CAD build for the part. Positions are in the model's coordinates, mm. Face numbers are marked on the shaded views. A direction names the side the tool comes from. Coordinates: 2 decimals unless noted, no trailing zeros. Loops run counter-clockwise (first coordinate to the right, second up) from the corner with the lowest first, then second, coordinate; pieces in that order, holes last. Notation, with made-up numbers: (-32, 43.25) -> (26, 43.25) arc R36 cw to (26, 79.25) -> close; hole circle Ø7 at (63, 77). An arc over 180 degrees is marked (long way). Write item = value, one per line. Start each with the question number.
(1) Drill centre lines: line 1 (Z direction, x = 3.25, y = 4); line 2 (Z direction, x = 20.5, y = 5.6); line 3 (Z direction, x = 21.25, y = 5.15). Where is each one in solid material? Low to high. Write a range as from..to.
(2) Pull direction Z, two halves, no side cores. Call the marked faces 4, 5 and 6: +Z half, -Z half, draft (parallel to the pull), parting line (faces both ways), or undercut.
(3) Band-saw the part on C-C (x = 11.5). Write the cut outline in (y, z).
(4) Band-saw the part on A-A (x = 5.25). Write the cut outline in (y, z), and give its area (3 significant figures).
(5) Band-saw the part on B-B (z = -2). Write the cut outline in (x, y).
(6) Flat gauge pins, fed straight in: P1, Ø1.8, axis at x = 4.5, y = 3.5, coming from the -Z side; P2, Ø1.8, axis at x = 11.5, z = -29, coming from the -Y side; P3, Ø0.8, axis at y = 3, z = -23.5, coming from the -X side. Where does each tip first touch, or does it go through?
(7) Tool access for the marked faces 1, 2 and 3: list every direction of +Z, -Z, +X, -X, +Y, -Y with a clear straight run to the whole face (end or side of a thin tool).
(8) Band-saw the part on D-D (z = -26). Write the cut outline in (x, y), and give its area (3 significant figures).
```python
from build123d import *

# Parameters (mm, degrees)
BOSS_EXTRUDE1_DEPTH = 6
SKETCH2_R           = 1
CUT_EXTRUDE1_DEPTH  = 40.862262856
SKETCH3_R           = 1
CUT_EXTRUDE2_DEPTH  = 40.862262856


with BuildPart() as part:
    # Sketch1 → Boss-Extrude1 (new body)
    with BuildSketch(Plane(origin=(0, 0, 0), x_dir=(1, 0, 0), z_dir=(0, 1, 0))):
        Polygon((0, 0), (0, 4), (6, 4), (6, 8), (0, 8), (0, 12), (6, 12), (6, 16), (0, 16), (0, 20), (6, 20), (6, 24), (0, 24), (0, 28), (6, 28), (6, 32), (23, 32), (23, 0), align=None)
    extrude(amount=BOSS_EXTRUDE1_DEPTH)

    # Sketch2 → Cut-Extrude1 (cut, through all)
    with BuildSketch(Plane(origin=(0, 6, 0), x_dir=(1, 0, 0), z_dir=(0, 1, 0))):
        with Locations(Location((2, 26, 0), (0, 0, 270))):
            Circle(SKETCH2_R)
        with Locations(Location((2, 18, 0), (0, 0, 270))):
            Circle(SKETCH2_R)
        with Locations(Location((2, 10, 0), (0, 0, 270))):
            Circle(SKETCH2_R)
        with Locations(Location((2, 2, 0), (0, 0, 270))):
            Circle(SKETCH2_R)
        with Locations((6, 22)):
            Circle(SKETCH2_R)
        with Locations((6, 30)):
            Circle(SKETCH2_R)
        with Locations((6, 14)):
            Circle(SKETCH2_R)
        with Locations((6, 6)):
            Circle(SKETCH2_R)
        with Locations(Location((21, 29, 0), (0, 0, 270))):
            Circle(SKETCH2_R)
        with Locations(Location((21, 9, 0), (0, 0, 270))):
            Circle(SKETCH2_R)
        with Locations(Location((17, 29, 0), (0, 0, 270))):
            Circle(SKETCH2_R)
        with Locations(Location((17, 9, 0), (0, 0, 270))):
            Circle(SKETCH2_R)
    extrude(amount=-CUT_EXTRUDE1_DEPTH, mode=Mode.SUBTRACT)

    # Sketch3 → Cut-Extrude2 (cut, through all)
    with BuildSketch(Plane(origin=(0, 6, 0), x_dir=(1, 0, 0), z_dir=(0, 1, 0))):
        with Locations(Location((11.5, 29, 0), (0, 0, 270))):
            Circle(SKETCH3_R)
        with Locations(Location((11.5, 26, 0), (0, 0, 270))):
            Circle(SKETCH3_R)
    extrude(amount=-CUT_EXTRUDE2_DEPTH, mode=Mode.SUBTRACT)


solid = part.part
```
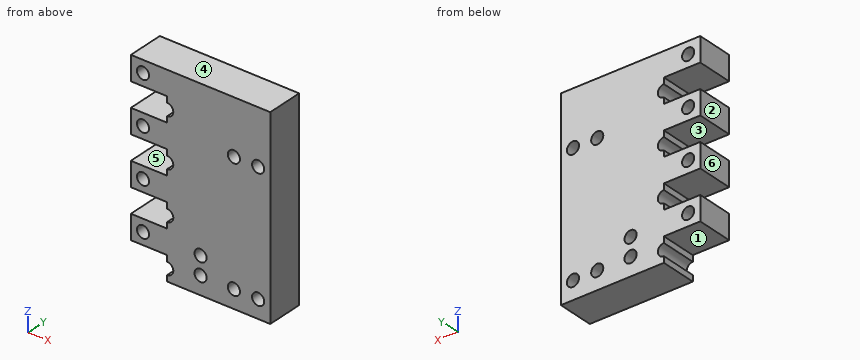
Findings below:
q1.line_1 = -28..-24, -20..-16, -12..-8, -4..0
q1.line_2 = -32..-29.87, -28.13..-9.87, -8.13..0
q1.line_3 = -32..-29.97, -28.03..-9.97, -8.03..0
q2.face_4 = +Z half
q2.face_5 = undercut
q2.face_6 = draft
q3.outline = (0, -32) -> (6, -32) -> (6, -30) -> (0, -30) -> close; (0, -28) -> (6, -28) -> (6, -27) -> (0, -27) -> close; (0, -25) -> (6, -25) -> (6, 0) -> (0, 0) -> close
q4.outline = (0, -28) -> (6, -28) -> (6, -24) -> (0, -24) -> close; (0, -20) -> (6, -20) -> (6, -16) -> (0, -16) -> close; (0, -12) -> (6, -12) -> (6, -8) -> (0, -8) -> close; (0, -4) -> (6, -4) -> (6, 0) -> (0, 0) -> close
q4.area = 96.0 mm²
q5.outline = (0, 0) -> (1, 0) -> (1, 6) -> (0, 6) -> close; (3, 0) -> (23, 0) -> (23, 6) -> (3, 6) -> close
q6.P1 = -28
q6.P2 = through
q6.P3 = 6
q7.face_1 = -Z, -X, +Y, -Y
q7.face_2 = +Z, -Z, -X, +Y, -Y
q7.face_3 = -X, +Y, -Y
q8.outline = (0, 0) -> (1, 0) -> (1, 6) -> (0, 6) -> close; (3, 0) -> (10.5, 0) -> (10.5, 6) -> (3, 6) -> close; (12.5, 0) -> (23, 0) -> (23, 6) -> (12.5, 6) -> close
q8.area = 114 mm²
